Design review of the part built by this model. Coordinates are the model's own, in mm. Coordinates: 2 decimals unless noted, no trailing zeros. Write each loop counter-clockwise with the first axis right and the second up, starting at its lowest first coordinate (ties: lowest second). Pieces come first, ordered by that corner, then holes. Notation, with made-up numbers: (21, 47.5) - (57, 47.5) arc R35 ccw to (57, 85.5) - close; hole circle Ø4 at (11, 75.5). An arc over 180 degrees is marked (long way). Answer as CSV lines item,"result". Start each with the question number.
Q1. Mouldability with a two-part tool opening along Z and no side actions: class faces 1 (the face through (-10, -3, -35)), 2 (the face through (36.949, -14.985, -0.66)), 3 (the face through (-20, -32, 10)) as pulls with the +Z half, pulls with the -Z half, needs draft (parallel to the pull), parting line crosses it, or undercut.
Q2. We need section C-C (x = -6.5). Write out the cut boundary in (y, z), plus the area to 3 significant figures.
Q3. For line 1 along X through (y, z) = (-12, -15.5); line 2 along Y through (x, z) = (39, 0); line 3 along Z through (x, y) = (35.5, 0), list the stretches that pass through material, from the lowest coordinate up. Write a range as [from, to].
Q4. We need section D-D (z = 17). Write out the cut boundary in (x, y), plus the area to 3 significant figures.
Q5. We need section A-A (y = 4). Write out the cut boundary in (x, z), plus the area to 3 significant figures.
Q6. We need section B-B (z = 0). Write out the cut boundary in (x, y), plus the area to 3 significant figures.
Q7. Clearance check with flat-ended pins moving along their axes: pin 1 (1.5 mm diameter, centred on y = -6, z = -3.5, fed in from -X); pin 2 (5 mm diameter, centred on x = 32, z = -25, fed in from +Y); pin 3 (4 mm diameter, centred on y = 11, z = 13.5, fed in from +X). State where each tip first meets the part, or that it passes through.
Autodesk Inventor part; units mm, degrees
ref_plane "YZ Plane" through (0, 0, 0) normal (1, 0, 0) x (0, 1, 0)
ref_plane "XZ Plane" through (0, 0, 0) normal (0, 1, 0) x (-1, 0, 0)
ref_plane "XY Plane" through (0, 0, 0) normal (0, 0, 1) x (1, 0, 0)
sketch "Эскиз1" plane through (0, 0, 0) normal (0, 1, 0) x (-1, 0, 0)
  arc A0 (-45, 0) -> (45, 0) centre (0, 0) ccw
  arc A1 (-35, 0) -> (35, 0) centre (0, 0) ccw
  line L0 (45, 0) -> (35, 0)
  line L1 (-35, 0) -> (-45, 0)
  line L2 (63, 0) -> (-63, 0)
  dimension "d0" = 45
  dimension "d1" = 35
revolve "Вращение1" add sketch "Эскиз1" angle 360 about axis through (-10, 0, 0) along (1, 0, 0) contours L1 A1 L0 A0
sketch "Эскиз2" plane through (0, 0, 0) normal (0, 1, 0) x (-1, 0, 0)
  line L0 (30, 10) -> (10, 10)
  line L1 (10, 10) -> (10, -45)
  line L2 (10, -45) -> (30, -45)
  line L3 (30, -45) -> (30, 10)
  line L4 (0, -87.9025) -> (0, 67.1504)
  line L5 (63, 0) -> (-63, 0)
  circle A0 centre (0, 0) radius 45
  dimension "d3" = 10
  dimension "d4" = 20
  dimension "d5" = 10
extrude "Выдавливание1" cut sketch "Эскиз2" along normal through all both and the other way through all contours L3 L5 L1 L0 | L3 A0 L1 L5 | L3 L2 L1 A0
sketch "Эскиз3" plane through (0, 0, 0) normal (1, 0, 0) x (0, 1, 0)
  circle A0 centre (0, 0) radius 15
  dimension "d8" = 30
extrude "Выдавливание2" cut sketch "Эскиз3" along normal through all
properties part number "Пирамида"
Results list:
1,face 1,"needs draft"
1,face 2,"undercut"
1,face 3,"pulls with the -Z half"
2,outline,"circle Ø89.06 at (0, 0); hole circle Ø68.78 at (0, 0)"
2,area,"2,510 mm2"
3,line 1,"x = [-40.51, -30], [29, 40.51]"
3,line 2,"y = [-22.45, -15], [15, 22.45]"
3,line 3,"z = [-27.65, -15], [15, 27.65]"
4,outline,"circle Ø83.33 at (0, 0); hole circle Ø61.19 at (0, 0)"
4,area,"2,510 mm2"
5,outline,"(-30, -33.3) - (-30, -17.58) arc R34.77 cw (long way) to (31.62, 14.46) - (42.43, 14.46) arc R44.82 ccw (long way) to start; (-10, -43.69) arc R44.82 ccw to (42.43, -14.46) - (31.62, -14.46) arc R34.77 cw to (-10, -33.3) - close"
5,area,"1,970 mm2"
6,outline,"(-30, -33.54) - (-30, -18.03) arc R35 cw to (-30, 18.03) - (-30, 33.54) arc R45 ccw to start; (-10, -43.87) arc R45 ccw to (42.43, -15) - (31.62, -15) arc R35 cw to (-10, -33.54) - close; (-10, 33.54) arc R35 cw to (31.62, 15) - (42.43, 15) arc R45 ccw to (-10, 43.87) - close"
6,area,"1,730 mm2"
7,pin 1,"stops at x = -44.57"
7,pin 2,"stops at y = 23.93"
7,pin 3,"stops at x = 42.28"
